Could you check a few things on this model? Use its own coordinates, in mm. A direction names the side the tool comes from. Round coordinates to 2 decimals unless told otherwise and drop trailing zeros. Loops run counter-clockwise (first coordinate to the right, second up) from the corner with the lowest first, then second, coordinate; pieces in that order, holes last. Notation, with made-up numbers: (-3, 58) -> (49, 58) arc R19 ccw to (49, 66) -> close; hole circle Ø6 at (-17, -20.75). An arc over 180 degrees is marked (long way). One line per item, written item: value.
from build123d import *

# Parameters (mm, degrees)
SZKIC1_R                    = 2.9
DODANIE_WYCI_GNI_CIE1_DEPTH = 26.7
DODANIE_WYCI_GNI_CIE2_START = 19.3
DODANIE_WYCI_GNI_CIE2_DEPTH = 1.5
DODANIE_WYCI_GNI_CIE3_DEPTH = 29.6
DODANIE_WYCI_GNI_CIE4_START = 29.6
SZKIC1_5_R                  = 2.9
DODANIE_WYCI_GNI_CIE4_DEPTH = 4
WYTNIJ_WYCI_GNI_CIE1_DEPTH  = 4
SZYK_KO_OWY1_COUNT          = 40
DODANIE_WYCI_GNI_CIE5_DEPTH = 4
ZAOKR_GLENIE1_R             = 0.5
SZKIC5_R                    = 0.5


with BuildPart() as part:
    # Szkic1 → Dodanie-wyci_gni_cie1 (new body)
    with BuildSketch(Plane(origin=(0, 0, 0), x_dir=(1, 0, 0), z_dir=(0, 1, 0))):
        with BuildLine():
            Line((-20.9, 6.6), (-20.9, -6.6))
            Line((-20.9, -6.6), (-7.4, -6.6))
            Line((-7.4, -6.6), (-7.4, -3.6))
            ThreePointArc((-7.4, -3.6), (-11, 0), (-7.4, 3.6))
            Line((-7.4, 3.6), (-7.4, 6.6))
            Line((-7.4, 6.6), (-20.9, 6.6))
        make_face()
        with BuildLine():
            Line((-7.4, -3.6), (-7.4, -6.6))
            Line((-7.4, -6.6), (7.1, -6.6))
            Line((7.1, -6.6), (7.1, 6.6))
            Line((7.1, 6.6), (-7.4, 6.6))
            Line((-7.4, 6.6), (-7.4, 3.6))
            ThreePointArc((-7.4, 3.6), (-11, 0), (-7.4, -3.6))
        make_face()
        Circle(SZKIC1_R, mode=Mode.SUBTRACT)
        Circle(SZKIC1_R)
    extrude(amount=DODANIE_WYCI_GNI_CIE1_DEPTH)

    # Szkic1_3 → Dodanie-wyci_gni_cie2 (add)
    with BuildSketch(Plane(origin=(0, 0, 0), x_dir=(1, 0, 0), z_dir=(0, 1, 0)).offset(DODANIE_WYCI_GNI_CIE2_START)):
        with BuildLine():
            Line((7.1, 6.6), (7.1, -6.6))
            Line((7.1, -6.6), (13.1, -6.6))
            Line((13.1, -6.6), (13.1, -1))
            Line((13.1, -1), (12.465564437, -1))
            ThreePointArc((12.465564437, -1), (8.2, 0), (12.465564437, 1))
            Line((12.465564437, 1), (13.1, 1))
            Line((13.1, 1), (13.1, 6.6))
            Line((13.1, 6.6), (7.1, 6.6))
        make_face()
        with BuildLine():
            Line((-26.9, -6.6), (-20.9, -6.6))
            Line((-20.9, -6.6), (-20.9, 6.6))
            Line((-20.9, 6.6), (-26.9, 6.6))
            Line((-26.9, 6.6), (-26.9, 1))
            Line((-26.9, 1), (-26.265564437, 1))
            ThreePointArc((-26.265564437, 1), (-22, 0), (-26.265564437, -1))
            Line((-26.265564437, -1), (-26.9, -1))
            Line((-26.9, -1), (-26.9, -6.6))
        make_face()
    extrude(amount=DODANIE_WYCI_GNI_CIE2_DEPTH)

    # Szkic1_4 → Dodanie-wyci_gni_cie3 (add)
    with BuildSketch(Plane(origin=(0, 0, 0), x_dir=(1, 0, 0), z_dir=(0, 1, 0))):
        with BuildLine():
            Line((-7.4, -3.6), (-7.4, -6.6))
            Line((-7.4, -6.6), (7.1, -6.6))
            Line((7.1, -6.6), (7.1, 6.6))
            Line((7.1, 6.6), (-7.4, 6.6))
            Line((-7.4, 6.6), (-7.4, 3.6))
            ThreePointArc((-7.4, 3.6), (-11, 0), (-7.4, -3.6))
        make_face()
    extrude(amount=DODANIE_WYCI_GNI_CIE3_DEPTH)

    # Szkic1_5 → Dodanie-wyci_gni_cie4 (add)
    with BuildSketch(Plane(origin=(0, 0, 0), x_dir=(1, 0, 0), z_dir=(0, 1, 0)).offset(DODANIE_WYCI_GNI_CIE4_START)):
        with Locations(Location((0, 0, 0), (0, 0, 270))):
            Circle(SZKIC1_5_R)
    extrude(amount=DODANIE_WYCI_GNI_CIE4_DEPTH)

    # Szkic3 → Wytnij-wyci_gni_cie1 (cut)
    with BuildSketch(Plane(origin=(0, 33.6, 0), x_dir=(1, 0, 0), z_dir=(0, 1, 0))):
        Polygon((-0.227531378, 2.891060268), (0, 2.66352889), (0.227531378, 2.891060268), (0.227531378, 3.66352889), (-0.227531378, 3.66352889), align=None)
    wytnij_wyci_gni_cie1 = extrude(amount=-WYTNIJ_WYCI_GNI_CIE1_DEPTH, mode=Mode.SUBTRACT)

    # Szyk ko_owy1: Wytnij-wyci_gni_cie1 ×40 about axis
    szyk_ko_owy1_axis = Axis((0, 0, 0), (0, 1, 0))
    for i in range(1, SZYK_KO_OWY1_COUNT):
        add(wytnij_wyci_gni_cie1.rotate(szyk_ko_owy1_axis, i * 360 / SZYK_KO_OWY1_COUNT), mode=Mode.SUBTRACT)

    # Szkic4 → Dodanie-wyci_gni_cie5 (add)
    with BuildSketch(Plane(origin=(7.1, 0, 0), x_dir=(0, 0, -1), z_dir=(1, 0, 0))):
        with BuildLine():
            Line((-2.5, 3), (2.5, 3))
            ThreePointArc((2.5, 3), (2.853553391, 3.146446609), (3, 3.5))
            Line((3, 3.5), (3, 5.5))
            ThreePointArc((3, 5.5), (2.853553391, 5.853553391), (2.5, 6))
            Line((2.5, 6), (-2.5, 6))
            ThreePointArc((-2.5, 6), (-2.853553391, 5.853553391), (-3, 5.5))
            Line((-3, 5.5), (-3, 3.5))
            ThreePointArc((-3, 3.5), (-2.853553391, 3.146446609), (-2.5, 3))
        make_face()
    extrude(amount=DODANIE_WYCI_GNI_CIE5_DEPTH)

    # Zaokr_glenie1
    zaokr_glenie1_edges = [part.edges().sort_by_distance(p)[0] for p in [
        (11.1, 5.853553391, -2.853553391),
        (11.1, 6, 0),
        (11.1, 5.853553391, 2.853553391),
        (11.1, 4.5, 3),
        (11.1, 3.146446609, 2.853553391),
        (11.1, 3, 0),
        (11.1, 3.146446609, -2.853553391),
        (11.1, 4.5, -3),
    ]]
    fillet(zaokr_glenie1_edges, radius=ZAOKR_GLENIE1_R)

    # Wyci_gni_cie po _cie_ce1: sweep along a path in Szkic6
    with BuildLine(Plane.XY) as wyci_gni_cie_po_cie_ce1_path:
        Line((11.1, 4.5), (13.1, 4.5))
        ThreePointArc((13.1, 4.5), (14.514213562, 3.914213562), (15.1, 2.5))
        Line((15.1, 2.5), (15.1, 0))
    # Szkic5 → Wyci_gni_cie po _cie_ce1 (sweep)
    with BuildSketch(Plane(origin=(11.1, 0, 0), x_dir=(0, 0, -1), z_dir=(1, 0, 0))):
        with Locations((-1.5, 4.5)):
            Circle(SZKIC5_R)
        with Locations((0, 4.5)):
            Circle(SZKIC5_R)
        with Locations((1.5, 4.5)):
            Circle(SZKIC5_R)
    sweep(path=wyci_gni_cie_po_cie_ce1_path.line)


solid = part.part
(1) For faces 1 (the face through (14.612, 1.232, 1.608)), 2 (the face through (-7.4, 28, 5)), 3 (the face through (11.1, 5, 1)), which set-ups out of +Z, -Z, +X, -X, +Y, -Y let a thin tool reach every point of the face, with its end or its side?
Recorded:
face 1: -Y
face 2: +Z, -X, +Y
face 3: none
(2) Thinking about a two-plate mould opening in X: for faces 4 (the face through (-7, 15, -6.6)), 5 (the face through (14.656, 1.232, -0.231)), 6 (the face through (-11, 28, 0)), which applies, released by +X, released by -X, zero draft, split by the parting line, or undercut?
Recorded:
face 4: zero draft
face 5: undercut
face 6: released by -X
(3) If we section it at B-B, the plane y = 2: Please give me the cut outline in (x, z), then the cut area to 3 significant figures.
Recorded:
outline: (-20.9, -6.6) -> (7.1, -6.6) -> (7.1, 6.6) -> (-20.9, 6.6) -> close; circle Ø1 at (15.1, -1.5); circle Ø1 at (15.1, 0); circle Ø1 at (15.1, 1.5)
area: 372 mm²
(4) If we section it at C-C, the plane z = 4.5: Please give me the cut outline in (x, y).
Recorded:
outline: (-26.9, 19.3) -> (-20.9, 19.3) -> (-20.9, 0) -> (7.1, 0) -> (7.1, 19.3) -> (13.1, 19.3) -> (13.1, 20.8) -> (7.1, 20.8) -> (7.1, 29.6) -> (-7.4, 29.6) -> (-7.4, 26.7) -> (-20.9, 26.7) -> (-20.9, 20.8) -> (-26.9, 20.8) -> close
(5) If we section it at D-D, the plane y = 20: Please give me the cut outline in (x, z).
Recorded:
outline: (-26.9, -6.6) -> (13.1, -6.6) -> (13.1, -1) -> (12.47, -1) arc R2.25 cw (long way) to (12.47, 1) -> (13.1, 1) -> (13.1, 6.6) -> (-26.9, 6.6) -> (-26.9, 1) -> (-26.27, 1) arc R2.25 cw (long way) to (-26.27, -1) -> (-26.9, -1) -> close
(6) If we section it at A-A, the plane x = -24.25: Please give me the cut outline in (y, z).
Recorded:
outline: (19.3, -6.6) -> (20.8, -6.6) -> (20.8, -2.25) -> (19.3, -2.25) -> close; (19.3, 2.25) -> (20.8, 2.25) -> (20.8, 6.6) -> (19.3, 6.6) -> close
(7) If I drill on L1, parallel to Z at x = 10.45, y = 20.5; L2, parallel to Y at x = 6, z = 5; L3, parallel to X at y = 20, z = -4.25, over which ranges is the centre line in solid material (lowest first)?
Recorded:
L1: -6.6 to -2.25, 2.25 to 6.6
L2: 0 to 29.6
L3: -26.9 to 13.1
(8) I'm going to push flat-ended pins straight in: pin 1 Ø2.5 at (y, z) = (28, -5) entering from -X; pin 2 Ø4 at (x, z) = (-13, -1) entering from +Y; pin 3 Ø5 at (x, z) = (9.5, -1.5) entering from +Y. Where does each tip first touch, or does it pass through?
Recorded:
pin 1: x = -7.4
pin 2: y = 26.7
pin 3: y = 29.6
